Work out the finished part from the listing and answer in its coordinate system (mm). A direction names the side the tool comes from. Round coordinates to 2 decimals unless told otherwise and drop trailing zeros. Loops run counter-clockwise (first coordinate to the right, second up) from the corner with the lowest first, then second, coordinate; pieces in that order, holes last. Notation, with made-up numbers: M 46.5,57.5 L 63.5,57.5 A32 cw 63.5,87.5 Z; hole C 13,-11 d8. An arc over 180 degrees is marked long. One line per item, written item: value.
```python
from build123d import *

# Parameters (mm, degrees)
PAD_DEPTH       = 30
POCKET_DEPTH    = 25.001
PAD003_DEPTH    = 12
PAD001_DEPTH    = 36
PAD002_DEPTH    = 12
SKETCH004_R     = 9
POCKET001_DEPTH = 36.001
FILLET_R        = 2


with BuildPart() as pad003:
    # Sketch → Pad (new body, symmetric)
    with BuildSketch(Plane.YZ):
        Polygon((0, 0), (-25, 0), (-25, 72), (-13, 72), (-13, 49), (0, 49), (0, 37), (-13, 37), (-13, 12), (0, 12), align=None)
    extrude(amount=PAD_DEPTH, both=True)

    # Sketch001 → Pocket (cut, through all)
    with BuildSketch(Plane(origin=(0, -25, 0), x_dir=(0, 0, -1), z_dir=(0, -1, 0))):
        with BuildLine():
            ThreePointArc((-17, 4.5), (-25, 12.5), (-33, 4.5))
            Line((-33, 4.5), (-33, -4.5))
            ThreePointArc((-33, -4.5), (-25, -12.5), (-17, -4.5))
            Line((-17, 4.5), (-17, -4.5))
        make_face()
    extrude(amount=-POCKET_DEPTH, mode=Mode.SUBTRACT)

    # Sketch005 → Pad003 (new body)
    with BuildSketch(Plane(origin=(-30, 0, 0), x_dir=(0, 1, 0), z_dir=(-1, 0, 0))):
        Polygon((-25, 0), (-36, -72), (-25, -72), align=None)
    extrude(amount=-PAD003_DEPTH)


with BuildPart() as fusion:
    # Sketch002 → Pad001 (new body)
    with BuildSketch(Plane.XZ):
        with BuildLine():
            Line((-30, 72), (30, 72))
            ThreePointArc((30, 72), (42.727922, 102.727922), (12, 90))
            Line((12, 84), (12, 90))
            Line((-12, 84), (12, 84))
            Line((-12, 84), (-12, 90))
            ThreePointArc((-12, 90), (-42.727922, 102.727922), (-30, 72))
        make_face()
    extrude(amount=PAD001_DEPTH)

    # Sketch003 → Pad002 (new body)
    with BuildSketch(Plane(origin=(0, 0, 0), x_dir=(1, 0, 0), z_dir=(0, 1, 0))):
        with BuildLine():
            ThreePointArc((-30, -72), (-48, -90), (-30, -108))
            Line((-30, -108), (30, -108))
            ThreePointArc((30, -108), (48, -90), (30, -72))
            Line((-30, -72), (30, -72))
        make_face()
    extrude(amount=-PAD002_DEPTH)

    # Sketch004 → Pocket001 (cut, through all)
    with BuildSketch(Plane.XZ.offset(36)):
        with Locations((30, 90)):
            Circle(SKETCH004_R)
        with Locations((-30, 90)):
            Circle(SKETCH004_R)
    extrude(amount=-POCKET001_DEPTH, mode=Mode.SUBTRACT)

    # Fillet
    fillet_edges = [fusion.edges().sort_by_distance(p)[0] for p in [
        (12, -24, 84),
        (0, -12, 84),
        (-12, -24, 84),
    ]]
    fillet(fillet_edges, radius=FILLET_R)

    # Fusion: union Pad003
    add(pad003.part)


solid = fusion.part
```
1) Each of these flat-tipped pins is pushed along its axis until it touches: pin 1 (1.2 mm diameter, centred on y = -29.5, z = 88.5, fed in from +X); pin 2 (20 mm diameter, centred on y = -6.5, z = 36.5, fed in from +X); pin 3 (5 mm diameter, centred on x = -34, y = -16, fed in from +Z). Where does it stop, or does it pass through?
Check values:
pin 1: x = 47.98
pin 2: x = 30
pin 3: z = 107.94
2) For faces 4 (the face through (-30, -18, 35)), 5 (the face through (-47.224, -17.748, 95.23)), 6 (the face through (0, -12, 99)), 7 (the face through (0, -13, 16)), 8 (the face through (-18, -28, 51)), determine the directions among +Z, -Z, +X, -X, +Y, -Y from which every point of the face is accessible in a straight line to the end or side of a thin tool.
Check values:
face 4: -Z, -X, +Y, -Y
face 5: -Y
face 6: +Z, -Y
face 7: +X, -X, +Y
face 8: -Z, +X, -Y
3) Find section D-D (y = -18). Give the vertices of the cut face in (x, z).
Check values:
outline: M -30,0 L 30,0 L 30,72 A18 ccw long 12,90 L 12,86 A2 cw 10,84 L -10,84 A2 cw -12,86 L -12,90 A18 ccw long -30,72 Z; hole C -30,90 d18; hole M -4.5,17 L 4.5,17 A8 ccw 4.5,33 L -4.5,33 A8 ccw Z; hole C 30,90 d18
4) Find section C-C (z = 27.5). Give the vertices of the cut face in (x, y).
Check values:
outline: M -30,-29.2 L -18,-29.2 L -18,-25 L -12.1,-25 L -12.1,-13 L -30,-13 Z; M 12.1,-25 L 30,-25 L 30,-13 L 12.1,-13 Z
5) Find section B-B (x = 0.5). Give the vertices of the cut face in (y, z).
Check values:
outline: M -36,72 L -25,72 L -25,33 L -13,33 L -13,37 L 0,37 L 0,49 L -13,49 L -13,72 L 0,72 L 0,108 L -12,108 L -12,86 A2 cw -14,84 L -36,84 Z; M -25,0 L 0,0 L 0,12 L -13,12 L -13,17 L -25,17 Z
6) Find the intervals of material crossed by probe 1 along Z at (x, y) = (-19.5, -7); probe 2 along Z at (x, y) = (30, -26); probe 3 along X at (y, z) = (-30, 54), in increasing order. Write a range as from..to.
Check values:
probe 1: 0..12, 37..49, 72..108
probe 2: 72..81, 99..108
probe 3: -30..-18
7) The mould has two halves that part along Z. Classify faces 1 (the face through (6, -30, 72)), 2 (the face through (28.049, -18.252, 81.214)), 3 (the face through (-1, 0, 90)): +Z half, -Z half, draft (parallel to the pull), parting line (faces both ways), or undercut.
Check values:
face 1: -Z half
face 2: undercut
face 3: draft
8) Find section A-A (y = -8.5). Give the vertices of the cut face in (x, z).
Check values:
outline: M -30,0 L 30,0 L 30,12 L -30,12 Z; M -30,37 L 30,37 L 30,49 L -30,49 Z; M -30,72 L 30,72 A18 ccw 30,108 L -30,108 A18 ccw Z; hole C -30,90 d18; hole C 30,90 d18
